Model file for the job. Use its own axes, mm. Face numbers are marked on the shaded views. Round coordinates to 2 decimals unless told otherwise and drop trailing zeros. Order: outer loops, then holes, each group sorted by start corner. A loop starts at its lowest first (then second) coordinate and runs counter-clockwise, first axis right, second up. Notation, with made-up numbers: (60.25, -16.5) -> (87.25, -16.5) arc R27 cw to (87.25, 20.5) -> close; hole circle Ø7 at (50.5, -39.5). An arc over 180 degrees is marked (long way). Use CSV: the item, a comma, the result in double quotes.
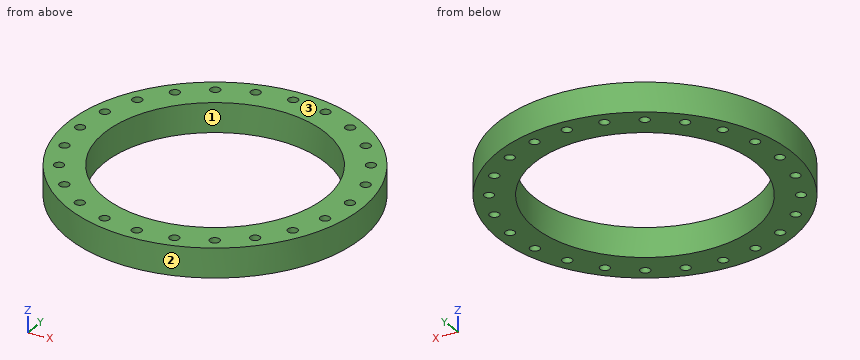
```python
from build123d import *

# Parameters (mm, degrees)
SKETCH1_R                   = 63.8302
SKETCH1_R_2                 = 48.0314
EXTRUDE1_DEPTH              = 12.7
F_19_0_166_DIAMETER_HOLE1_D = 4.2164
CIRPATTERN1_COUNT           = 24


with BuildPart() as part:
    # Sketch1 → Extrude1 (new body)
    with BuildSketch(Plane.XY):
        Circle(SKETCH1_R)
        Circle(SKETCH1_R_2, mode=Mode.SUBTRACT)
    extrude(amount=EXTRUDE1_DEPTH)

    # #19 (0.166) Diameter Hole1 (through all)
    with Locations(Plane(origin=(0, 57.8612, 12.7), x_dir=(1, 0, 0), z_dir=(0, 0, 1))):
        with Locations((0, 0)):
            f_19_0_166_diameter_hole1 = Hole(F_19_0_166_DIAMETER_HOLE1_D / 2)

    # CirPattern1: #19 (0.166) Diameter Hole1 ×24 about axis
    cirpattern1_axis = Axis((0, 0, 0), (0, 0, 1))
    for i in range(1, CIRPATTERN1_COUNT):
        add(f_19_0_166_diameter_hole1.rotate(cirpattern1_axis, i * 360 / CIRPATTERN1_COUNT), mode=Mode.SUBTRACT)


solid = part.part
```
Q1. Mould opens along X. For the marked faces 1, 2 and 3 say: +X half, -X half, draft (parallel to the pull), parting line (faces both ways), or undercut.
From the geometry:
face 1,"undercut"
face 2,"parting line"
face 3,"draft"
Q2. Cut at C-C (y = 22.5). Give the cut face in (x, z).
From the geometry:
outline,"(-59.73, 0) -> (-42.44, 0) -> (-42.44, 12.7) -> (-59.73, 12.7) -> close; (42.44, 0) -> (59.73, 0) -> (59.73, 12.7) -> (42.44, 12.7) -> close"
Q3. Pin check, flat tips, straight feed: pin 1 (6.5 mm diameter, centred on x = 14.98, y = -55.89, fed in from -Z); pin 2 (3 mm diameter, centred on y = 16.5, z = 2.5, fed in from +X); pin 3 (3 mm diameter, centred on y = 28.5, z = 4, fed in from +X); pin 4 (3 mm diameter, centred on x = -50.5, z = 5, fed in from -Y). Stop position of each tip, or through.
From the geometry:
pin 1,"stops at z = 0"
pin 2,"stops at x = 62.04"
pin 3,"stops at x = 57.84"
pin 4,"stops at y = -40.91"
Q4. Cut at A-A (y = 0). Give the cut face in (x, z), plus the area to 3 significant figures.
From the geometry:
outline,"(-63.83, 0) -> (-59.97, 0) -> (-59.97, 12.7) -> (-63.83, 12.7) -> close; (-55.75, 0) -> (-48.03, 0) -> (-48.03, 12.7) -> (-55.75, 12.7) -> close; (48.03, 0) -> (55.75, 0) -> (55.75, 12.7) -> (48.03, 12.7) -> close; (59.97, 0) -> (63.83, 0) -> (63.83, 12.7) -> (59.97, 12.7) -> close"
area,"294 mm²"
Q5. Cut at D-D (z = 3.25). State how many separate pieces and enclosed holes the cut face has, plus the area to 3 significant figures.
From the geometry:
separate pieces,"1"
enclosed holes,"25"
area,"5,220 mm²"
Q6. Probe line 1 along Y through (x, z) = (0, 6); line 2 along X through (y, z) = (48.5, 9.5); line 3 along X through (y, z) = (-16.5, 1). List the from-to ranges inside material, lowest first.
From the geometry:
line 1,"y = -63.83 to -59.97, -55.75 to -48.03, 48.03 to 55.75, 59.97 to 63.83"
line 2,"x = -41.5 to -30.29, -27.57 to 27.57, 30.29 to 41.5"
line 3,"x = -61.66 to -57.35, -54.43 to -45.11, 45.11 to 54.43, 57.35 to 61.66"
